```python
from build123d import *

# Parameters (mm, degrees)
BOSS_EXTRUDE1_DEPTH  = 27.5
SKETCH4_R            = 8.1
CUT_EXTRUDE1_DEPTH   = 67.638952573
M5_CLEARANCE_HOLE1_D = 5.5
SKETCH7_W            = 30
SKETCH7_H            = 15
CUT_EXTRUDE2_DEPTH   = 67.191011474
FILLET1_R            = 5


with BuildPart() as part:
    # Sketch1 → Boss-Extrude1 (new, symmetric)
    with BuildSketch(Plane(origin=(0, 0, 0), x_dir=(1, 0, 0), z_dir=(0, 1, 0))):
        Polygon((0, 0), (0, 40), (3.5, 40), (3.5, 3.5), (48.5, 3.5), (48.5, 0), align=None)
    extrude(amount=BOSS_EXTRUDE1_DEPTH, both=True)

    # Sketch4 → Cut-Extrude1 (cut, through all)
    with BuildSketch(Plane(origin=(0, 0, -3.5), x_dir=(-1, 0, 0), z_dir=(0, 0, -1))):
        with Locations((-26, 10)):
            Circle(SKETCH4_R)
    extrude(amount=-CUT_EXTRUDE1_DEPTH, mode=Mode.SUBTRACT)

    # M5 Clearance Hole1 (through all)
    with Locations(Plane.ZY):
        with Locations((-10.5, -17.5), (-33, -17.5)):
            Hole(M5_CLEARANCE_HOLE1_D / 2)

    # Sketch7 → Cut-Extrude2 (cut, through all)
    with BuildSketch(Plane(origin=(3.5, 0, 0), x_dir=(0, 0, -1), z_dir=(1, 0, 0))):
        with Locations((25, 20)):
            Rectangle(SKETCH7_W, SKETCH7_H)
    extrude(amount=-CUT_EXTRUDE2_DEPTH, mode=Mode.SUBTRACT)

    # Fillet1
    fillet1_edges = [part.edges().sort_by_distance(p)[0] for p in [
        (1.75, 12.5, -40),
        (1.75, 12.5, -10),
        (1.75, 27.5, -10),
        (1.75, -27.5, -40),
        (48.5, -27.5, -1.75),
        (48.5, 27.5, -1.75),
    ]]
    fillet(fillet1_edges, radius=FILLET1_R)


solid = part.part
```
Design review of the part built by this model. Coordinates are the model's own, in mm. A direction names the side the tool comes from. Round coordinates to 2 decimals unless told otherwise and drop trailing zeros. Write each loop counter-clockwise with the first axis right and the second up, starting at its lowest first coordinate (ties: lowest second). Pieces come first, ordered by that corner, then holes. Notation, with made-up numbers: (-35.5, 31.25) -> (-26.5, 31.25) arc R19 cw to (-26.5, 37.25) -> close; hole circle Ø3 at (84, 85.5). An arc over 180 degrees is marked (long way). Write item = value, one per line. Start each with the question number.
1) Mouldability with a two-part tool opening along Y and no side actions: class faces 1 (the face through (3.5, -6, -22)), 2 (the face through (1.73, 14, -11.43)), 3 (the face through (1.775, -17.379, -30.253)) as +Y half, -Y half, draft (parallel to the pull), parting line (faces both ways), or undercut.
2) Tool access review of faces 4 (the face through (2, 20, -10)), 5 (the face through (26, 0, -3.5)), 6 (the face through (47, -26.07, -1.73)): name each direction out of +Z, -Z, +X, -X, +Y, -Y from which nothing blocks a thin tool from reaching the whole face with its end or side.
3) Clearance check with flat-ended pins moving along their axes: pin 1 (9 mm diameter, centred on y = -17.5, z = -10.5, fed in from +X); pin 2 (2 mm diameter, centred on x = 20.5, y = 7, fed in from +Z); pin 3 (9 mm diameter, centred on y = -17.5, z = -33, fed in from -X); pin 4 (4 mm diameter, centred on x = 12.5, y = -17.5, fed in from -Z). State where each tip first meets the part, or that it passes through.
4) Wall thickness on probe 1 along Y at (x, z) = (1, -33); probe 2 along X at (y, z) = (9.5, -2.5); probe 3 along Z at (x, y) = (37.5, 19): over which ranges is each line inside the solid? List them lowest first. Write a range as from..to.
5) Take a section at A-A, the plane z = -33. State the section outline as (x, y) points.
6) Take a section at B-B, the plane x = 25.5. State the section outline as (y, z) points.
7) Take a section at C-C, the plane y = -2.5. State the section outline as (x, z) points.
8) Take a section at D-D, the plane y = 16.5. State the section outline as (x, z) points, plus the area to 3 significant figures.
Results list:
q1.face_1 = draft
q1.face_2 = +Y half
q1.face_3 = undercut
q2.face_4 = -Z, +X, -X, +Y
q2.face_5 = -Z, +X, +Y, -Y
q2.face_6 = +Z, -Z, +X, -Y
q3.pin_1 = 3.5
q3.pin_2 = through
q3.pin_3 = 0
q3.pin_4 = -3.5
q4.probe_1 = -27.5..-20.25, -14.75..12.5
q4.probe_2 = 0..17.92, 34.08..48.5
q4.probe_3 = -3.5..0
q5.outline = (0, -27.5) -> (3.5, -27.5) -> (3.5, -20.25) -> (0, -20.25) -> close; (0, -14.75) -> (3.5, -14.75) -> (3.5, 12.5) -> (0, 12.5) -> close
q6.outline = (-27.5, -3.5) -> (1.92, -3.5) -> (1.92, 0) -> (-27.5, 0) -> close; (18.08, -3.5) -> (27.5, -3.5) -> (27.5, 0) -> (18.08, 0) -> close
q7.outline = (0, -40) -> (3.5, -40) -> (3.5, -3.5) -> (48.5, -3.5) -> (48.5, 0) -> (0, 0) -> close
q8.outline = (0, -10.1) -> (3.5, -10.1) -> (3.5, -3.5) -> (21.17, -3.5) -> (21.17, 0) -> (0, 0) -> close; (30.83, -3.5) -> (48.5, -3.5) -> (48.5, 0) -> (30.83, 0) -> close
q8.area = 159 mm²
